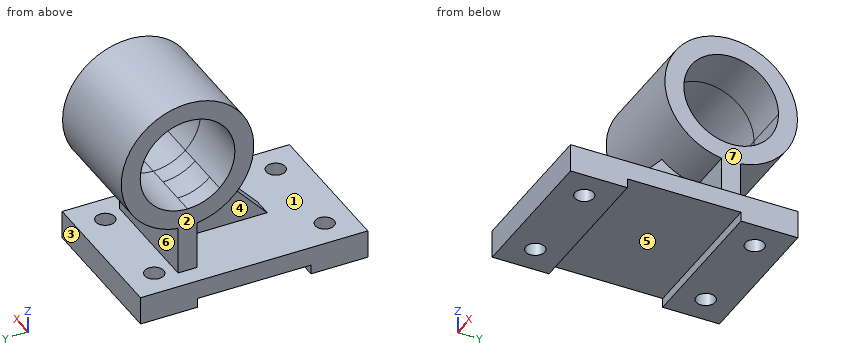
from build123d import *

# Parameters (mm, degrees)
F1_DEPTH      = 10
F3_DEPTH      = 25
F3_DEPTH_BACK = 35
F4_DEPTH      = 25
F5_W          = 80
F5_H          = 120
F5_W_2        = 10
F5_H_2        = 55
F6_DEPTH      = 15
F8_DEPTH      = 60
F9_W          = 60
F9_H          = 5
F10_DEPTH     = 80
F11_R         = 5
F12_DEPTH     = 51.887460053


with BuildPart() as f1:
    # F0 (on Right) → F1 (new body)
    with BuildSketch(Plane.YZ):
        Polygon((0, 0), (0, 60), (-55, 0), align=None)
    extrude(amount=F1_DEPTH)

    # F2 (on face) → F3 (join, two sides)
    with BuildSketch(Plane.YZ.offset(10)) as f3_sk:
        with BuildLine():
            ThreePointArc((0, 25), (24.7487373415, 35.2512626585), (35, 60))
            ThreePointArc((35, 60), (-14.0932134389, 92.0371867518), (-23.6503619981, 34.199605093))
            Line((-23.6503619981, 34.199605093), (-16.8931157129, 41.571146495))
            ThreePointArc((-16.8931157129, 41.571146495), (-10.0665810278, 82.8837048227), (25, 60))
            ThreePointArc((25, 60), (17.6776695297, 42.3223304703), (0, 35))
            Line((0, 35), (0, 25))
        make_face()
        with BuildLine():
            Line((-16.8931157129, 41.571146495), (-23.6503619981, 34.199605093))
            ThreePointArc((-23.6503619981, 34.199605093), (-12.688305211, 27.3808812064), (0, 25))
            Line((0, 25), (0, 35))
            ThreePointArc((0, 35), (-9.0630751507, 36.7006294331), (-16.8931157129, 41.571146495))
        make_face()
    extrude(amount=F3_DEPTH)
    extrude(f3_sk.sketch, amount=-F3_DEPTH_BACK)

    # F4 (cut): a face of the model
    f4_faces = [f1.faces().sort_by_distance(p)[0] for p in [
        (10, -5.9044146652, 44.8209197235),
    ]]
    extrude(f4_faces, amount=-F4_DEPTH, mode=Mode.SUBTRACT)

    # F5 (on face) → F6 (join)
    with BuildSketch(Plane(origin=(0, 0, 0), x_dir=(1, 0, 0), z_dir=(0, 0, -1))):
        with Locations((5, 30)):
            Rectangle(F5_W, F5_H)
        with Locations((5, 27.5)):
            Rectangle(F5_W_2, F5_H_2, mode=Mode.SUBTRACT)
        with Locations((5, 27.5)):
            Rectangle(F5_W_2, F5_H_2)
    extrude(amount=F6_DEPTH)

    # F7 (on face) → F8 (join, through all)
    with BuildSketch(Plane.YZ.offset(35)):
        with BuildLine():
            ThreePointArc((5, 25.3589838486), (0, 25), (-5, 25.3589838486))
            Line((-5, 25.3589838486), (-5, -0.8262397959))
            Line((-5, -0.8262397959), (-5, -1.0180029073))
            Line((-5, -1.0180029073), (5, -1.0180029073))
            Line((5, -1.0180029073), (5, 25.3589838486))
        make_face()
    extrude(amount=-F8_DEPTH)

    # F9 (on face) → F10 (cut)
    with BuildSketch(Plane.YZ.offset(45)):
        with Locations((-30, -12.5)):
            Rectangle(F9_W, F9_H)
    extrude(amount=-F10_DEPTH, mode=Mode.SUBTRACT)

    # F11 (on face) → F12 (cut)
    with BuildSketch(Plane.XY):
        with Locations((-20, -75)):
            Circle(F11_R)
        with Locations((30, -75)):
            Circle(F11_R)
        with Locations((30, 15)):
            Circle(F11_R)
        with Locations((-20, 15)):
            Circle(F11_R)
    extrude(amount=-F12_DEPTH, mode=Mode.SUBTRACT)


solid = f1.part
Could you check a few things on this model? Use its own coordinates, in mm. Face numbers are marked on the shaded views. A direction names the side the tool comes from. Round coordinates to 2 decimals unless told otherwise and drop trailing zeros. Order: outer loops, then holes, each group sorted by start corner. A loop starts at its lowest first (then second) coordinate and runs counter-clockwise, first axis right, second up.
(1) Which directions (+Z, -Z, +X, -X, +Y, -Y) give clear straight access to the entire face, cutting with the end or side of a thin tool? Please do the marked faces 1, 2, 3 and 4.
Response values:
face 1: none
face 2: +Z, -X, +Y, -Y
face 3: -Z, +X, -X, +Y
face 4: -X, -Y
(2) Please list where these lines run through material, in increasing order: line 1 along Y through (x, z) = (30, -8); line 2 along Z through (x, y) = (16.5, 18); line 3 along X through (y, z) = (-29, 77).
Response values:
line 1: y = -90 to -80, -70 to 10, 20 to 30
line 2: z = -15 to 0, 29.98 to 42.65, 77.35 to 90.02
line 3: x = -25 to 35
(3) Imagine slicing it at A-A (x = 30). Write out the boundary of the cut face in (y, z).
Response values:
outline: (-90, -15) - (-80, -15) - (-80, 0) - (-90, 0) - close; (-70, -15) - (-60, -15) - (-60, -10) - (0, -10) - (0, -15) - (10, -15) - (10, 0) - (5, 0) - (5, 25.36) arc R35 ccw (long way) to (-5, 25.36) - (-5, 0) - (-70, 0) - close; (20, -15) - (30, -15) - (30, 0) - (20, 0) - close; hole circle Ø50 at (0, 60)
(4) Imagine slicing it at C-C (x = -11). Write out the boundary of the cut face in (y, z).
Response values:
outline: (-90, -15) - (-60, -15) - (-60, -10) - (0, -10) - (0, -15) - (30, -15) - (30, 0) - (5, 0) - (5, 25.36) arc R35 ccw (long way) to (-5, 25.36) - (-5, 0) - (-90, 0) - close; hole circle Ø50 at (0, 60)
(5) Imagine slicing it at D-D (z = -1.5). Write out the boundary of the cut face in (x, y).
Response values:
outline: (-35, -90) - (45, -90) - (45, 30) - (-35, 30) - close; hole circle Ø10 at (-20, -75); hole circle Ø10 at (-20, 15); hole circle Ø10 at (30, -75); hole circle Ø10 at (30, 15)
(6) Imagine slicing it at B-B (y = -75). Write out the boundary of the cut face in (x, z).
Response values:
outline: (-35, -15) - (-25, -15) - (-25, 0) - (-35, 0) - close; (-15, -15) - (25, -15) - (25, 0) - (-15, 0) - close; (35, -15) - (45, -15) - (45, 0) - (35, 0) - close
(7) If we mould it in two halves opening along Z, with no side actions, what happens to the marked faces 5, 6 and 7? For each: released by +Z, released by -Z, zero draft, split by the parting line, or undercut.
Response values:
face 5: released by -Z
face 6: undercut
face 7: zero draft
(8) I'm going to push flat-ended pins straight in: pin 1 (1.5 mm diameter, centred on x = 19.5, z = -13.5, fed in from +Y); pin 2 (9 mm diameter, centred on x = 30, y = 15, fed in from +Z); pin 3 (6 mm diameter, centred on x = -8.5, y = -20.5, fed in from -Z); pin 4 (6 mm diameter, centred on y = 14, z = 73.5, fed in from -X). Where does each tip first touch, or does it pass through?
Response values:
pin 1: stops at y = 30
pin 2: stops at z = 93.39
pin 3: stops at z = -10
pin 4: passes through
